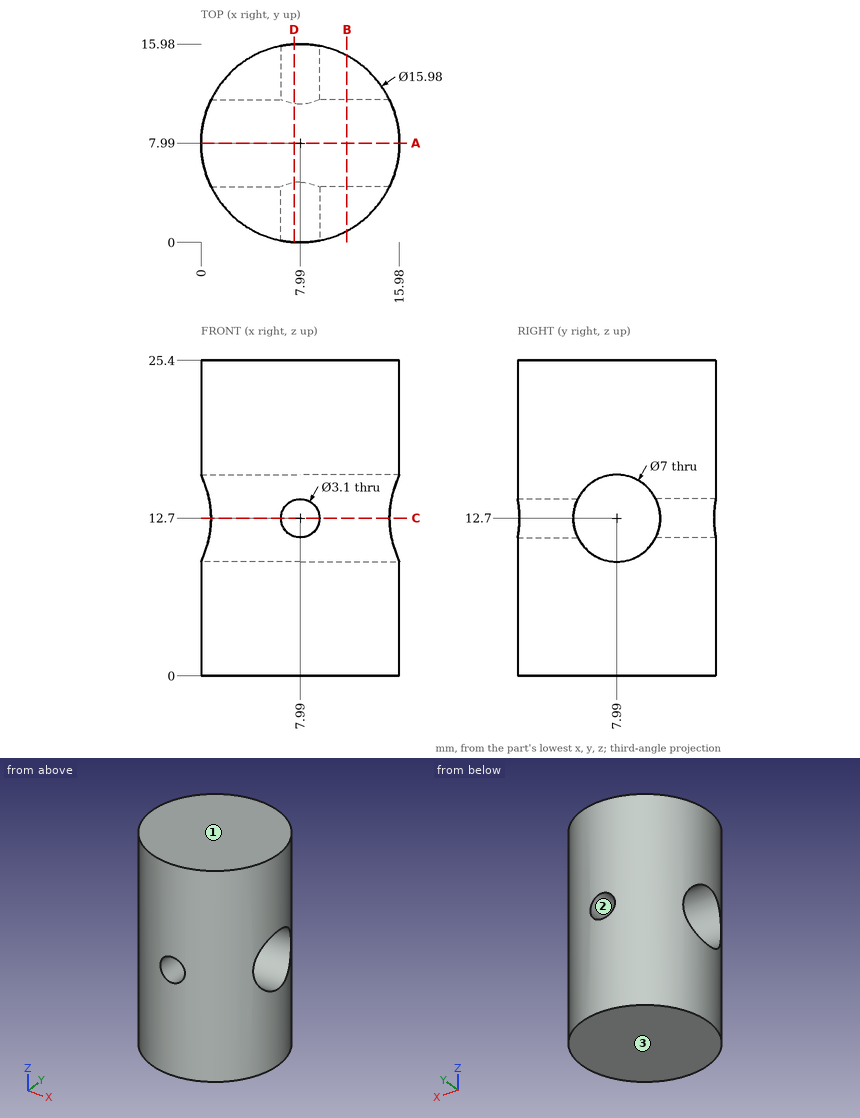
Part print with two shaded views. Sizes in mm from the minimum x, y, z corner. Give positions to 0.01 mm unless a question says otherwise; leave off trailing zeros. Order: outer loops, then holes, each group sorted by start corner. A loop starts at its lowest first (then second) coordinate and runs counter-clockwise, first axis right, second up. Notation, with made-up numbers: M 65,3.5 L 77,3.5 A28 ccw 77,26.5 Z; hole C 31.25,3 d3. An arc over 180 degrees is marked long. Put each result on its own line as item: value.
Item 1: Cut at C-C on z = 12.7. Write the cut outline in (x, y).
Results are:
outline: M 0.81,4.49 A7.99 ccw 6.44,0.15 L 6.44,4.49 Z; M 0.81,11.49 L 6.44,11.49 L 6.44,15.83 A7.99 ccw Z; M 9.54,0.15 A7.99 ccw 15.17,4.49 L 9.54,4.49 Z; M 9.54,11.49 L 15.17,11.49 A7.99 ccw 9.54,15.83 Z
Item 2: Cut at A-A on y = 7.99. Write the cut outline in (x, z).
Results are:
outline: M 0,0 L 15.98,0 L 15.98,9.2 L 0,9.2 Z; M 0,16.2 L 15.98,16.2 L 15.98,25.4 L 0,25.4 Z
Item 3: Wall check: probe 1 along Z at (x, y) = (7.99, 2.2); probe 2 along Y at (x, z) = (3, 12.7); probe 3 along Z at (x, y) = (10, 9). Give the ranges that are in metal, low to high.
Results are:
probe 1: 0 to 11.15, 14.25 to 25.4
probe 2: 1.75 to 4.49, 11.49 to 14.23
probe 3: 0 to 9.35, 16.05 to 25.4
Item 4: Cut at D-D on x = 7.5. Write the cut outline in (y, z), then the cut area to 3 significant figures.
Results are:
outline: M 0.02,0 L 15.96,0 L 15.96,11.23 L 11.17,11.23 A3.5 cw 4.81,11.23 L 0.02,11.23 Z; M 0.02,14.17 L 4.81,14.17 A3.5 cw 11.17,14.17 L 15.96,14.17 L 15.96,25.4 L 0.02,25.4 Z
area: 340 mm2
Item 5: Cut at B-B on x = 11.75. Write the cut outline in (y, z).
Results are:
outline: M 0.94,0 L 15.04,0 L 15.04,25.4 L 0.94,25.4 Z; hole C 7.99,12.7 d7
Item 6: Pull direction Z, two halves, no side cores. Call the marked faces 1, 2 and 3: +Z half, -Z half, draft (parallel to the pull), parting line (faces both ways), or undercut.
Results are:
face 1: +Z half
face 2: undercut
face 3: -Z half
